from build123d import *

# Parameters (mm, degrees)
SKETCH1_W           = 279.4
SKETCH1_H           = 279.4
BOSS_EXTRUDE1_DEPTH = 5.715
CUT_EXTRUDE4_REACH  = 199.648
SKETCH6_R           = 5.0419
CUT_EXTRUDE6_REACH  = 199.648
FILLET1_R           = 5.08


with BuildPart() as part:
    # Sketch1 → Boss-Extrude1 (new body)
    with BuildSketch(Plane(origin=(0, 0, 0), x_dir=(1, 0, 0), z_dir=(0, 1, 0))):
        Rectangle(SKETCH1_W, SKETCH1_H)
    extrude(amount=BOSS_EXTRUDE1_DEPTH)

    # Sketch6 → Cut-Extrude4 (cut, up to next)
    with BuildSketch(Plane(origin=(0, 5.715, 0), x_dir=(1, 0, 0), z_dir=(0, 1, 0)), mode=Mode.PRIVATE) as cut_extrude4_sk1:
        with Locations(Location((-114.3, 114.3, 0), (0, 0, 270))):
            Circle(SKETCH6_R)
    cut_extrude4_tool1 = extrude(cut_extrude4_sk1.sketch, amount=-CUT_EXTRUDE4_REACH, mode=Mode.PRIVATE) & part.part
    # Sketch6 → Cut-Extrude4 (cut, up to next)
    with BuildSketch(Plane(origin=(0, 5.715, 0), x_dir=(1, 0, 0), z_dir=(0, 1, 0)), mode=Mode.PRIVATE) as cut_extrude4_sk2:
        with Locations(Location((114.3, 114.3, 0), (0, 0, 270))):
            Circle(SKETCH6_R)
    cut_extrude4_tool2 = extrude(cut_extrude4_sk2.sketch, amount=-CUT_EXTRUDE4_REACH, mode=Mode.PRIVATE) & part.part
    # Sketch6 → Cut-Extrude4 (cut, up to next)
    with BuildSketch(Plane(origin=(0, 5.715, 0), x_dir=(1, 0, 0), z_dir=(0, 1, 0)), mode=Mode.PRIVATE) as cut_extrude4_sk3:
        with Locations(Location((114.3, -114.3, 0), (0, 0, 270))):
            Circle(SKETCH6_R)
    cut_extrude4_tool3 = extrude(cut_extrude4_sk3.sketch, amount=-CUT_EXTRUDE4_REACH, mode=Mode.PRIVATE) & part.part
    # Sketch6 → Cut-Extrude4 (cut, up to next)
    with BuildSketch(Plane(origin=(0, 5.715, 0), x_dir=(1, 0, 0), z_dir=(0, 1, 0)), mode=Mode.PRIVATE) as cut_extrude4_sk4:
        with Locations(Location((-114.3, -114.3, 0), (0, 0, 270))):
            Circle(SKETCH6_R)
    cut_extrude4_tool4 = extrude(cut_extrude4_sk4.sketch, amount=-CUT_EXTRUDE4_REACH, mode=Mode.PRIVATE) & part.part
    add(cut_extrude4_tool1.solids().sort_by_distance((-114.3, 5.715, -114.3))[0], mode=Mode.SUBTRACT)
    add(cut_extrude4_tool2.solids().sort_by_distance((114.3, 5.715, -114.3))[0], mode=Mode.SUBTRACT)
    add(cut_extrude4_tool3.solids().sort_by_distance((114.3, 5.715, 114.3))[0], mode=Mode.SUBTRACT)
    add(cut_extrude4_tool4.solids().sort_by_distance((-114.3, 5.715, 114.3))[0], mode=Mode.SUBTRACT)

    # Sketch8 → Cut-Extrude6 (cut, up to next)
    with BuildSketch(Plane(origin=(0, 5.715, 0), x_dir=(1, 0, 0), z_dir=(0, 1, 0)), mode=Mode.PRIVATE) as cut_extrude6_sk1:
        with BuildLine():
            Line((-139.7, 139.7), (-139.7, 124.46))
            Line((-139.7, 124.46), (-121.739487758, 106.499487758))
            ThreePointArc((-121.739487758, 106.499487758), (-106.499487758, 106.499487758), (-106.499487758, 121.739487758))
            Line((-106.499487758, 121.739487758), (-124.46, 139.7))
            Line((-124.46, 139.7), (-139.7, 139.7))
        make_face()
    cut_extrude6_tool1 = extrude(cut_extrude6_sk1.sketch, amount=-CUT_EXTRUDE6_REACH, mode=Mode.PRIVATE) & part.part
    # Sketch8 → Cut-Extrude6 (cut, up to next)
    with BuildSketch(Plane(origin=(0, 5.715, 0), x_dir=(1, 0, 0), z_dir=(0, 1, 0)), mode=Mode.PRIVATE) as cut_extrude6_sk2:
        with BuildLine():
            Line((-124.46, -139.7), (-106.499487758, -121.739487758))
            ThreePointArc((-106.499487758, -121.739487758), (-106.499487758, -106.499487758), (-121.739487758, -106.499487758))
            Line((-121.739487758, -106.499487758), (-139.7, -124.46))
            Line((-139.7, -124.46), (-139.7, -139.7))
            Line((-139.7, -139.7), (-124.46, -139.7))
        make_face()
    cut_extrude6_tool2 = extrude(cut_extrude6_sk2.sketch, amount=-CUT_EXTRUDE6_REACH, mode=Mode.PRIVATE) & part.part
    # Sketch8 → Cut-Extrude6 (cut, up to next)
    with BuildSketch(Plane(origin=(0, 5.715, 0), x_dir=(1, 0, 0), z_dir=(0, 1, 0)), mode=Mode.PRIVATE) as cut_extrude6_sk3:
        with BuildLine():
            Line((139.7, -139.7), (139.7, -124.46))
            Line((139.7, -124.46), (121.739487758, -106.499487758))
            ThreePointArc((121.739487758, -106.499487758), (106.499487758, -106.499487758), (106.499487758, -121.739487758))
            Line((106.499487758, -121.739487758), (124.46, -139.7))
            Line((124.46, -139.7), (139.7, -139.7))
        make_face()
    cut_extrude6_tool3 = extrude(cut_extrude6_sk3.sketch, amount=-CUT_EXTRUDE6_REACH, mode=Mode.PRIVATE) & part.part
    # Sketch8 → Cut-Extrude6 (cut, up to next)
    with BuildSketch(Plane(origin=(0, 5.715, 0), x_dir=(1, 0, 0), z_dir=(0, 1, 0)), mode=Mode.PRIVATE) as cut_extrude6_sk4:
        with BuildLine():
            Line((124.46, 139.7), (106.499487758, 121.739487758))
            ThreePointArc((106.499487758, 121.739487758), (106.499487758, 106.499487758), (121.739487758, 106.499487758))
            Line((121.739487758, 106.499487758), (139.7, 124.46))
            Line((139.7, 124.46), (139.7, 139.7))
            Line((139.7, 139.7), (124.46, 139.7))
        make_face()
    cut_extrude6_tool4 = extrude(cut_extrude6_sk4.sketch, amount=-CUT_EXTRUDE6_REACH, mode=Mode.PRIVATE) & part.part
    add(cut_extrude6_tool1.solids().sort_by_distance((-122.047436, 5.715, -122.047436))[0], mode=Mode.SUBTRACT)
    add(cut_extrude6_tool2.solids().sort_by_distance((-122.047436, 5.715, 122.047436))[0], mode=Mode.SUBTRACT)
    add(cut_extrude6_tool3.solids().sort_by_distance((122.047436, 5.715, 122.047436))[0], mode=Mode.SUBTRACT)
    add(cut_extrude6_tool4.solids().sort_by_distance((122.047436, 5.715, -122.047436))[0], mode=Mode.SUBTRACT)

    # Fillet1
    fillet1_edges = [part.edges().sort_by_distance(p)[0] for p in [
        (124.46, 2.8575, -139.7),
        (139.7, 2.8575, -124.46),
        (139.7, 2.8575, 124.46),
        (124.46, 2.8575, 139.7),
        (-124.46, 2.8575, 139.7),
        (-139.7, 2.8575, 124.46),
        (-124.46, 2.8575, -139.7),
        (-139.7, 2.8575, -124.46),
    ]]
    fillet(fillet1_edges, radius=FILLET1_R)


solid = part.part
Geometry: final body of the model. Coordinates: model frame, mm. A direction names the side the tool comes from. Give positions to 0.01 mm unless a question says otherwise; leave off trailing zeros. Write each loop counter-clockwise with the first axis right and the second up, starting at its lowest first coordinate (ties: lowest second). Pieces come first, ordered by that corner, then holes. Notation, with made-up numbers: M -25.75,-36.75 L 25.25,-36.75 A25 ccw 25.25,0.25 Z; hole C 53,-7 d10. An arc over 180 degrees is marked long. Answer in a Markdown table with one row per item. Add a question column.
(1) Mould query, pull axis Z, two halves, no side actions, for faces 1 (the flat face through (-126.45, 2.9, -111.21)), 2 (the cylindrical face through (106.67, 2.9, 106.33)), 3 (the flat face through (-126.32, 2.9, 111.08)). Classes: +Z half, -Z half, draft (parallel to the pull), parting line (faces both ways), or undercut.
(2) Section A-A on y = 4.55. Return loops of the section in (x, z), and give its area (3 significant figures).
(3) Reachability of faces 4 (the flat face through (111.08, 2.9, 126.32)), 5 (the cylindrical face through (-106.33, 2.9, 106.67)), 6 (the flat face through (126.32, 2.9, -111.08)), 7 (the flat face through (126.45, 2.9, 111.21)), 8 (the flat face through (-111.21, 2.9, 126.45)) from +Z, -Z, +X, -X, +Y, -Y: full face, straight path, thin tool, end or side. Return the list, or none.
(4) Ray query, line 1 (Z direction, x = 110, y = 3.35); line 2 (X direction, y = 3.5, z = 107.5); line 3 (Z direction, x = -126.5, y = 5.5). Return the intervals inside material, ascending.
Result set:
| question | item | result |
|---|---|---|
| 1 | face 1 | -Z half |
| 1 | face 2 | undercut |
| 1 | face 3 | +Z half |
| 2 | outline | M -139.7,-112.2 A5.08 ccw -131.03,-115.79 L -121.74,-106.5 A10.78 cw -106.5,-121.74 L -115.79,-131.03 A5.08 ccw -112.2,-139.7 L 112.2,-139.7 A5.08 ccw 115.79,-131.03 L 106.5,-121.74 A10.78 cw 121.74,-106.5 L 131.03,-115.79 A5.08 ccw 139.7,-112.2 L 139.7,112.2 A5.08 ccw 131.03,115.79 L 121.74,106.5 A10.78 cw 106.5,121.74 L 115.79,131.03 A5.08 ccw 112.2,139.7 L -112.2,139.7 A5.08 ccw -115.79,131.03 L -106.5,121.74 A10.78 cw -121.74,106.5 L -131.03,115.79 A5.08 ccw -139.7,112.2 Z |
| 2 | area | 74,400 mm^2 |
| 3 | face 4 | +X, +Y, -Y |
| 3 | face 5 | +Y, -Y |
| 3 | face 6 | -Z, +Y, -Y |
| 3 | face 7 | +Z, +Y, -Y |
| 3 | face 8 | -X, +Y, -Y |
| 4 | line 1 | z = -139.7 to -125.24, -104.16 to 104.16, 125.24 to 139.7 |
| 4 | line 2 | x = -139.7 to -122.74, -105.62 to 105.62, 122.74 to 139.7 |
| 4 | line 3 | z = -111.26 to 111.26 |
